```python
from build123d import *

# Parameters (mm, degrees)
CROQUIS1_R                         = 10
SALIENTE_EXTRUIR1_DEPTH            = 20
CROQUIS2_R                         = 25
SALIENTE_EXTRUIR2_DEPTH            = 50
SALIENTE_EXTRUIR2_TAPER            = 20
CROQUIS3_R                         = 4
CORTAR_EXTRUIR2_DEPTH              = 70
TALADRO_DE_MARGEN_PARA_1_41_REACH  = 76.055
TALADRO_DE_MARGEN_PARA_1_41_BORE_R = 3.3782


with BuildPart() as part:
    # Croquis1 → Saliente-Extruir1 (new body)
    with BuildSketch(Plane(origin=(0, 0, 0), x_dir=(0, 0, -1), z_dir=(1, 0, 0))):
        Circle(CROQUIS1_R)
    extrude(amount=SALIENTE_EXTRUIR1_DEPTH)

    # Croquis2 → Saliente-Extruir2 (add)
    with BuildSketch(Plane(origin=(20, 0, 0), x_dir=(0, 0, -1), z_dir=(1, 0, 0))):
        Circle(CROQUIS2_R)
    extrude(amount=SALIENTE_EXTRUIR2_DEPTH, taper=SALIENTE_EXTRUIR2_TAPER)

    # Croquis3 → Cortar-Extruir2 (cut)
    with BuildSketch(Plane(origin=(70, 0, 0), x_dir=(0, 0, -1), z_dir=(1, 0, 0))):
        Circle(CROQUIS3_R)
    extrude(amount=-CORTAR_EXTRUIR2_DEPTH, mode=Mode.SUBTRACT)

    # Taladro de margen para 1/41 bore (on position points) → Taladro de margen para 1/41 (cut, up to next)
    with BuildSketch(Plane(origin=(10, 9.974931901, -0.707625302), x_dir=(0, 0.070762530204, 0.997493190112), z_dir=(0, 0.997493190112, -0.070762530204)), mode=Mode.PRIVATE) as taladro_de_margen_para_1_41_sk1:
        Circle(TALADRO_DE_MARGEN_PARA_1_41_BORE_R)
    taladro_de_margen_para_1_41_tool1 = extrude(taladro_de_margen_para_1_41_sk1.sketch, amount=-TALADRO_DE_MARGEN_PARA_1_41_REACH, mode=Mode.PRIVATE) & part.part
    add(taladro_de_margen_para_1_41_tool1.solids().sort_by_distance((10, 9.974932, -0.707625))[0], mode=Mode.SUBTRACT)


solid = part.part
```
Geometry check sheet. Reference: the model listing, model coordinates, mm. A direction names the side the tool comes from. Coordinates: 2 decimals unless noted, no trailing zeros. Loops run counter-clockwise (first coordinate to the right, second up) from the corner with the lowest first, then second, coordinate; pieces in that order, holes last.
Item 1: Release check for a two-part mould opening along Z. For faces 1 (the face through (0, -4.3, 0.1)), 2 (the face through (9.86, -9.76, 2.17)), 3 (the face through (35.49, -3.905, 0.867)) record: released by +Z, released by -Z, zero draft, split by the parting line, or undercut.
Item 2: Access from +Z, -Z, +X, -X, +Y, -Y to the whole of each face (thin tool, end or side, straight path). Record for faces 4 (the face through (20, -11, 0)), 5 (the face through (70, -3, -3)).
Item 3: Thickness scan on line 1 (Y direction, x = 50, z = 0); line 2 (Z direction, x = 24, y = -3.5); line 3 (Y direction, x = 21, z = 0). Record the ranges inside material, lowest first.
Item 4: Sectioned sample at A-A, the plane z = 0. Count the separate pieces of the cut face and the enclosed holes in it, then the cut area to 3 significant figures.
Item 5: Sectioned sample at C-C, the plane x = 39.5. Record the boundary of the cut face in (y, z), then the cut area to 3 significant figures.
Item 6: Go/stop test with flat-tipped pins: pin 1 Ø5 at (x, y) = (14.5, 13.5) entering from -Z; pin 2 Ø1.5 at (x, y) = (29.5, 10.5) entering from -Z; pin 3 Ø5 at (x, z) = (46, -16.5) entering from -Y; pin 4 Ø6 at (y, z) = (-14, 2) entering from -X. Record where each tip stops, or that it passes through.
Item 7: Sectioned sample at B-B, the plane x = 54. Record the boundary of the cut face in (y, z), then the cut area to 3 significant figures.
Check result:
1. face 1: zero draft
1. face 2: split by the parting line
1. face 3: undercut
2. face 4: -X
2. face 5: +Z, -Z, +X, +Y, -Y
3. line 1: y = -14.08 to -4, 4 to 14.08
3. line 2: z = -23.28 to -1.94, 1.94 to 23.28
3. line 3: y = -24.64 to -4, 4 to 24.64
4. separate pieces: 3
4. enclosed holes: 0
4. area: 1,390 mm2
5. outline: circle Ø35.81 at (0, 0); hole circle Ø8 at (0, 0)
5. area: 957 mm2
6. pin 1: passes through
6. pin 2: stops at z = -19.32
6. pin 3: stops at y = -7.14
6. pin 4: stops at x = 20
7. outline: circle Ø25.25 at (0, 0); hole circle Ø8 at (0, 0)
7. area: 450 mm2
